Check sheet for the modelled part. Datum: model origin and axes. Units: mm. Face numbers are marked on the shaded views. A direction names the side the tool comes from. Coordinates: 2 decimals unless noted, no trailing zeros. Loops run counter-clockwise (first coordinate to the right, second up) from the corner with the lowest first, then second, coordinate; pieces in that order, holes last. Notation, with made-up numbers: (-33, 63.25) - (-16, 63.25) arc R18 cw to (-16, 93.25) - close; hole circle Ø11 at (32, 67.25). An arc over 180 degrees is marked (long way). Write each question's results on one line, items separated by ' | '. Start each with the question number.
1. Cross-section at D-D (z = 1.5). Record the cut outline in (x, y), and give its area (3 significant figures).
2. Tool access check on the marked faces 4 and 5. Record the directions out of +Z, -Z, +X, -X, +Y, -Y that give a thin tool (end or side, any length) a straight path to the whole face; none if there is none.
3. Draft check along Y on the marked faces 1, 2 and 3. Enter one of: released by +Y, released by -Y, zero draft, split by the parting line, or undercut.
4. Gauge pin test, flat end, axial feed: P1, Ø9, axis at x = 2.5, y = 4, coming from the -Z side. Record the tip position at first contact, or that the pin passes through.
5. Cross-section at A-A (y = 25). Record the cut outline in (x, z).
6. Thickness scan on line 1 (X direction, y = 19.5, z = 8.75); line 2 (Z direction, x = 9.25, y = 14.5); line 3 (X direction, y = 34, z = 6.25). Record the ranges inside material, lowest first. Write a range as [from, to].
7. Cross-section at B-B (z = 6). Record the cut outline in (x, y), and give its area (3 significant figures).
8. Cross-section at C-C (x = 0). Record the cut outline in (y, z).
```python
from build123d import *

# Parameters (mm, degrees)
F1_DEPTH = 9
F3_DEPTH = 3
F4_R     = 2.1
F5_DEPTH = 38.001
F6_W     = 10
F6_H     = 15
F7_DEPTH = 9.001


with BuildPart() as f1:
    # F0 (on Top) → F1 (new body)
    with BuildSketch(Plane.XY):
        with BuildLine():
            Line((-15, 38), (-15, 0))
            Line((-15, 0), (-6.25, 0))
            ThreePointArc((-6.25, 0), (0, 6.25), (6.25, 0))
            Line((6.25, 0), (12, 0))
            Line((12, 0), (12, 38))
            Line((12, 38), (-15, 38))
        make_face()
    extrude(amount=F1_DEPTH)

    # F2 (on face) → F3 (cut)
    with BuildSketch(Plane(origin=(0, 0, 0), x_dir=(1, 0, 0), z_dir=(0, 0, -1))):
        with BuildLine():
            ThreePointArc((6.25, 0), (0, -6.25), (-6.25, 0))
            Line((-6.25, 0), (-8.25, 0))
            ThreePointArc((-8.25, 0), (0, -8.25), (8.25, 0))
            Line((8.25, 0), (6.25, 0))
        make_face()
    extrude(amount=-F3_DEPTH, mode=Mode.SUBTRACT)

    # F4 (on Front) → F5 (cut, through all)
    with BuildSketch(Plane.XZ):
        with Locations((-9.25, 6)):
            Circle(F4_R)
        with Locations((9.25, 6)):
            Circle(F4_R)
    extrude(amount=-F5_DEPTH, mode=Mode.SUBTRACT)

    # F6 (on face) → F7 (cut, through all)
    with BuildSketch(Plane.XY.offset(9)):
        with Locations((0, 22.395955)):
            Rectangle(F6_W, F6_H)
    extrude(amount=-F7_DEPTH, mode=Mode.SUBTRACT)


solid = f1.part
```
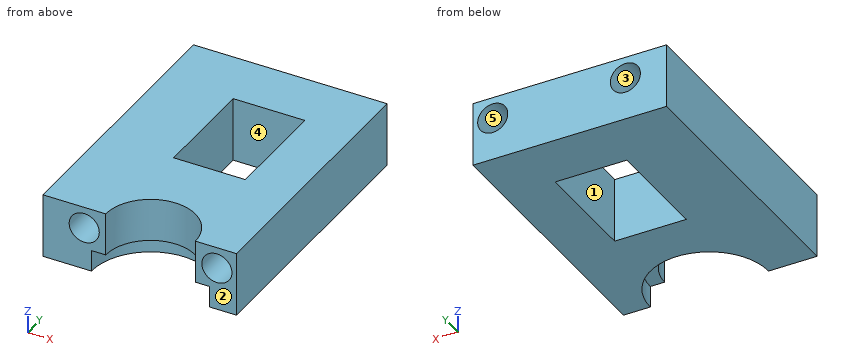
Established:
1) outline: (-15, 0) - (-8.25, 0) arc R8.25 cw to (8.25, 0) - (12, 0) - (12, 38) - (-15, 38) - close; hole (-5, 14.9) - (5, 14.9) - (5, 29.9) - (-5, 29.9) - close | area: 769 mm^2
2) face 4: +Z, -Z | face 5: +Y, -Y
3) face 1: undercut | face 2: released by -Y | face 3: zero draft
4) P1: z = 0
5) outline: (-15, 0) - (-5, 0) - (-5, 9) - (-15, 9) - close; (5, 0) - (12, 0) - (12, 9) - (5, 9) - close; hole circle Ø4.2 at (-9.25, 6); hole circle Ø4.2 at (9.25, 6)
6) line 1: [-15, -5], [5, 12] | line 2: [0, 3.9], [8.1, 9] | line 3: [-15, -11.34], [-7.16, 7.16], [11.34, 12]
7) outline: (-15, 0) - (-11.35, 0) - (-11.35, 38) - (-15, 38) - close; (-7.15, 0) - (-6.25, 0) arc R6.25 cw to (6.25, 0) - (7.15, 0) - (7.15, 38) - (-7.15, 38) - close; (11.35, 0) - (12, 0) - (12, 38) - (11.35, 38) - close; hole (-5, 14.9) - (5, 14.9) - (5, 29.9) - (-5, 29.9) - close | area: 495 mm^2
8) outline: (6.25, 3) - (8.25, 3) - (8.25, 0) - (14.9, 0) - (14.9, 9) - (6.25, 9) - close; (29.9, 0) - (38, 0) - (38, 9) - (29.9, 9) - close
